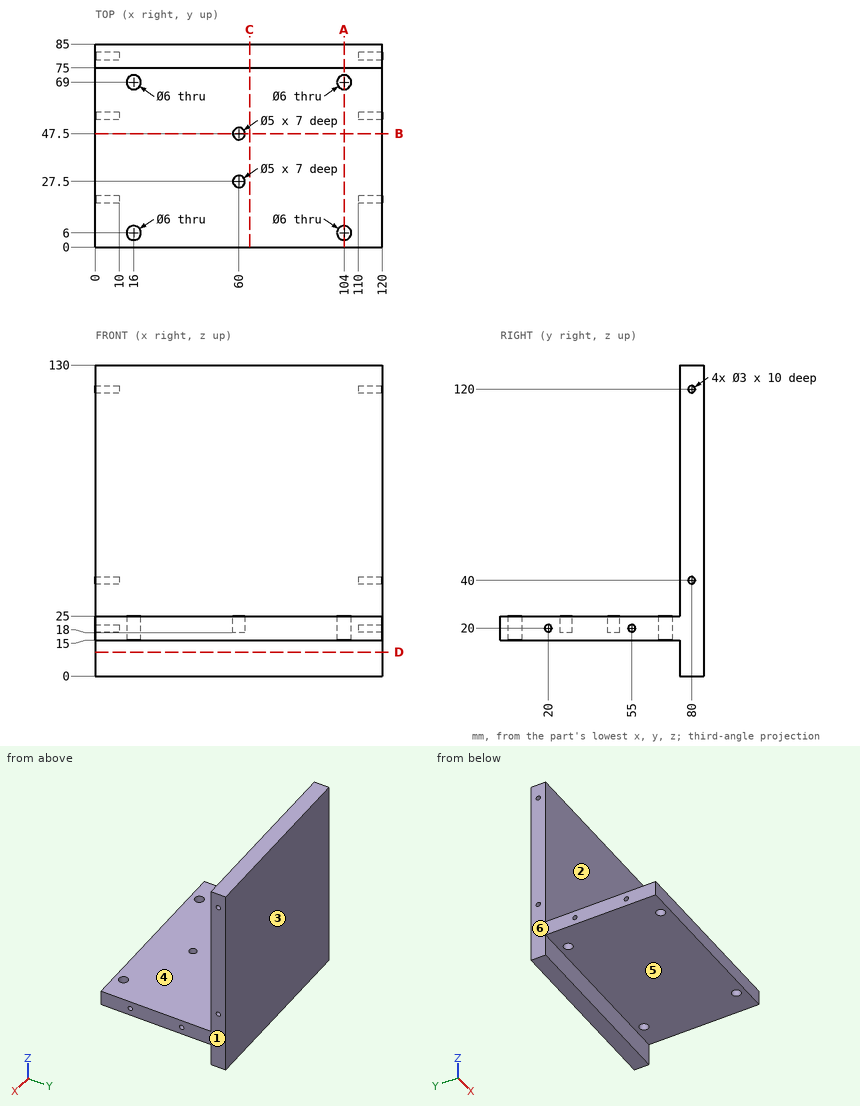
Verification items for this drawing (mm, ordinates from the low corner). A direction names the side the tool comes from. Give positions to 0.01 mm unless a question says otherwise; leave off trailing zeros. Write each loop counter-clockwise with the first axis right and the second up, starting at its lowest first coordinate (ties: lowest second). Pieces come first, ordered by that corner, then holes. Notation, with made-up numbers: (-11.75, 66.5) -> (22.25, 66.5) arc R13 ccw to (22.25, 80.5) -> close; hole circle Ø3 at (3.5, 12.5). An arc over 180 degrees is marked (long way). Use CSV: the item, a comma, the result in double quotes. Start each with the question number.
Q1. Cross-section at C-C on x = 64.5. Enter the section's corners in (y, z), and give its area (3 significant figures).
Q2. Cross-section at B-B on y = 47.5. Enter the section's corners in (x, z), and give its area (4 significant figures).
Q3. Tool access check on the marked faces 4, 5 and 6. Record the directions out of +Z, -Z, +X, -X, +Y, -Y that give a thin tool (end or side, any length) a straight path to the whole face; none if there is none.
Q4. Cross-section at A-A on x = 104. Enter the section's corners in (y, z).
Q5. Cross-section at D-D on z = 10. Enter the section's corners in (x, y), and give its area (3 significant figures).
Q6. Depth check by flat-ended pin: P1, Ø8, axis at x = 60, y = 27.5, coming from the +Z side; P2, Ø2.5, axis at x = 60, y = 48.5, coming from the +Z side; P3, Ø4.5, axis at x = 67.5, z = 9.5, coming from the -Y side. Enter the tip coordinate at first touch or a pass-through.
Q7. Release check for a two-part mould opening along Y. For the marked faces 1, 2 and 3 record: +Y half, -Y half, draft (parallel to the pull), parting line (faces both ways), or undercut.
Q8. Scan lines: line 1 along Z through (x, y) = (112, 80); line 2 along Y through (x, z) = (60, 22.75); line 3 along Z through (x, y) = (6.5, 55). Record each from-to range of solid material in increasing order.
Working result:
1,outline,"(0, 15) -> (75, 15) -> (75, 0) -> (85, 0) -> (85, 130) -> (75, 130) -> (75, 25) -> (0, 25) -> close"
1,area,"2,050 mm^2"
2,outline,"(0, 15) -> (120, 15) -> (120, 25) -> (62.5, 25) -> (62.5, 18) -> (57.5, 18) -> (57.5, 25) -> (0, 25) -> close"
2,area,"1,165 mm^2"
3,face 4,"+Z, +X, -X, -Y"
3,face 5,"-Z, +X, -X, -Y"
3,face 6,"+Z, -Z, -X, +Y, -Y"
4,outline,"(0, 15) -> (3, 15) -> (3, 25) -> (0, 25) -> close; (9, 15) -> (66, 15) -> (66, 25) -> (9, 25) -> close; (72, 15) -> (75, 15) -> (75, 0) -> (85, 0) -> (85, 130) -> (75, 130) -> (75, 25) -> (72, 25) -> close"
5,outline,"(0, 75) -> (120, 75) -> (120, 85) -> (0, 85) -> close"
5,area,"1,200 mm^2"
6,P1,"stops at z = 25"
6,P2,"stops at z = 18"
6,P3,"stops at y = 75"
7,face 1,"draft"
7,face 2,"-Y half"
7,face 3,"+Y half"
8,line 1,"z = 0 to 38.5, 41.5 to 118.5, 121.5 to 130"
8,line 2,"y = 0 to 25, 30 to 45, 50 to 85"
8,line 3,"z = 15 to 18.5, 21.5 to 25"
